CAD build for the part. Positions are in the model's coordinates, mm. A direction names the side the tool comes from. Round coordinates to 2 decimals unless told otherwise and drop trailing zeros. Order: outer loops, then holes, each group sorted by start corner. A loop starts at its lowest first (then second) coordinate and runs counter-clockwise, first axis right, second up. Notation, with made-up numbers: (81.5, -32) -> (93.5, -32) arc R31 ccw to (93.5, -1) -> close; hole circle Ø4 at (68.5, 47). An arc over 180 degrees is marked (long way). Return JSON: item names as keys, results as strings. Group by question number.
Q1. Which spindle directions (+Z, -Z, +X, -X, +Y, -Y) get a long thin tool onto all of the face, cutting with end or side? Do faces 4 (the flat face through (-31.18, -9, 2)), 5 (the flat face through (-31.18, 3, 5)), 6 (the flat face through (-37, 7.69, 5)). Say none if no direction does.
Q2. Cut at C-C (x = -12.5). Write the cut outline in (y, z), then the cut area to 3 significant figures.
Q3. Cut at D-D (y = -19). Write the cut outline in (x, z), then the cut area to 3 significant figures.
Q4. Cut at A-A (y = -3.5). Write the cut outline in (x, z).
Q5. Mould opens along X. For faces 1 (the flat face through (49.58, 22, 5)), 2 (the flat face through (24, 23, 9.35)), 3 (the flat face through (-2, 39.74, 3)) say: +X half, -X half, draft (parallel to the pull), parting line (faces both ways), or undercut.
Q6. Probe line 1 along X through (y, z) = (3, 4.75); line 2 along X through (y, z) = (6, 7); line 3 along X through (y, z) = (-5.5, 0.75). List the from-to ranges inside material, lowest first.
Q7. Flat gauge pins, fed straight in: pin 1 (5 mm diameter, centred on x = -64.5, z = 4, fed in from +Y); pin 2 (19 mm diameter, centred on x = -20.5, y = -2, fed in from +Z); pin 3 (1.6 mm diameter, centred on x = -10.5, z = 1, fed in from -Y). Where does each tip first touch, or does it go through?
Autodesk Inventor part; units mm, degrees
ref_plane "YZ Plane" through (0, 0, 0) normal (1, 0, 0) x (0, 1, 0)
ref_plane "XZ Plane" through (0, 0, 0) normal (0, 1, 0) x (-1, 0, 0)
ref_plane "XY Plane" through (0, 0, 0) normal (0, 0, 1) x (1, 0, 0)
sketch "Sketch1" plane through (0, 0, 0) normal (0, 0, 1) x (1, 0, 0)
  line L0 (0, 0) -> (49.58, 0)
  line L1 (49.58, 0) -> (49.58, 44.9)
  line L2 (49.58, 44.9) -> (0, 44.9)
  line L3 (0, 44.9) -> (0, 0)
  line L4 (49.58, 2.33) -> (27.13, 2.33)
  line L5 (27.13, 2.33) -> (27.13, 0)
  line L6 (27.13, 44.9) -> (27.13, 42.57)
  line L7 (27.13, 42.57) -> (49.58, 42.57)
  dimension "d0" = 49.58
  dimension "d1" = 44.9
  dimension "d2" = 22.45
  dimension "d3" = 2.33
extrude "Extrusion1" add sketch "Sketch1" along normal blind 9.35 contours L3 L2 L6 L7 L1 L4 L5 L0
sketch "Sketch2" plane through (0, 0, 0) normal (-1, 0, 0) x (0, 0, 1)
  line L0 (0, 44.9) -> (0, 0)
  line L1 (9.35, 44.9) -> (9.35, 0)
  line L2 (0, 44.9) -> (9.35, 44.9)
  line L3 (0, 39.74) -> (9.35, 39.74)
  line L4 (9.35, 39.74) -> (9.35, 7.69)
  line L5 (9.35, 7.69) -> (0, 7.69)
  line L6 (0, 7.69) -> (0, 39.74)
  dimension "d6" = 32.05
  dimension "d7" = 5.16
extrude "Extrusion2" add sketch "Sketch2" along normal blind 31.18 contours L3 L1 L5 L0
sketch "Sketch3" plane through (0, 0, 9.35) normal (0, 0, 1) x (1, 0, 0)
  line L0 (0, 39.74) -> (-31.18, 39.74)
  line L1 (-3.12, 39.74) -> (0, 39.74)
  line L2 (0, 39.74) -> (0, 7.69)
  line L3 (0, 7.69) -> (-3.12, 7.69)
  line L4 (-3.12, 7.69) -> (-3.12, 39.74)
extrude "Extrusion3" cut sketch "Sketch3" against normal blind 3.12
sketch "Sketch4" plane through (-31.18, 39.74, 0) normal (0, 1, 0) x (1, 0, 0)
  line L0 (0, -9.35) -> (0, 0)
  line L1 (28.06, -9.35) -> (0, -9.35)
  line L2 (31.18, 0) -> (0, 0)
  line L3 (28.06, -9.35) -> (0, -9.35)
  line L4 (0, -9.35) -> (0, 0)
  line L5 (0, 0) -> (28.06, 0)
  line L6 (28.06, 0) -> (28.06, -9.35)
extrude "Extrusion4" add sketch "Sketch4" along normal blind 6.86
sketch "Sketch5" plane through (-31.18, 7.69, 0) normal (0, -1, 0) x (1, 0, 0)
  line L0 (28.06, 0) -> (0, 0)
  line L1 (28.06, 9.35) -> (28.06, 0)
  line L2 (0, 0) -> (28.06, 0)
  line L3 (28.06, 0) -> (28.06, 3.12)
  line L4 (28.06, 3.12) -> (0, 3.12)
  line L5 (0, 3.12) -> (0, 0)
  dimension "d14" = 3.12
extrude "Extrusion5" add sketch "Sketch5" along normal blind 24.01
sketch "Sketch6" plane through (-31.18, 7.69, 3.12) normal (0, 0, 1) x (1, 0, 0)
  line L0 (0, 0) -> (9.35, 0)
  line L1 (9.35, 0) -> (9.35, -9.35)
  line L2 (9.35, -9.35) -> (0, -9.35)
  line L3 (0, -9.35) -> (0, 0)
  point P0 (31.18, -7.69)
  dimension "d17" = 9.35
  dimension "d18" = 9.35
extrude "Extrusion6" add sketch "Sketch6" along normal blind 3.12
sketch "Sketch7" plane through (-31.18, 0, 0) normal (-1, 0, 0) x (0, 0, 1)
  line L0 (3.12, 7.69) -> (0, 7.69)
  line L1 (3.12, -1.66) -> (0, -1.66)
  line L2 (0, -1.66) -> (0, 7.69)
  line L3 (0, 7.69) -> (3.12, 7.69)
  line L4 (3.12, 7.69) -> (3.12, -1.66)
  line L5 (0, 7.69) -> (6.24, 7.69)
  line L6 (6.24, 7.69) -> (6.24, 35.13)
  line L7 (6.24, 35.13) -> (0, 35.13)
  line L8 (0, 35.13) -> (0, 7.69)
  line L9 (0, -16.32) -> (0, 46.6)
  point P0 (0, 0)
  dimension "d21" = 27.44
  dimension "d24" = 6.24
extrude "Extrusion7" add sketch "Sketch7" along normal blind 12.47
sketch "Sketch8" plane through (-31.18, 35.13, 6.24) normal (0, 1, 0) x (1, 0, 0)
  line L0 (-12.47, 0) -> (-12.47, 6.24)
  line L1 (0, 6.24) -> (-12.47, 6.24)
  line L2 (0, 0) -> (-12.47, 0)
  line L3 (0, 6.24) -> (-3.12, 6.24)
  line L4 (-3.12, 6.24) -> (-3.12, 0)
  line L5 (-3.12, 0) -> (0, 0)
  line L6 (0, 0) -> (0, 6.24)
  point P0 (31.18, 6.24)
  dimension "d25" = 3.12
extrude "Extrusion8" cut sketch "Sketch8" against normal blind 6.24 contours L0 L1 L4 L2
sketch "Sketch9" plane through (-43.65, 0, 0) normal (-1, 0, 0) x (0, 0, 1)
  line L0 (0, 28.89) -> (0, -1.66)
  line L1 (0, 28.58) -> (9.35, 28.58)
  line L2 (9.35, 28.58) -> (9.35, -1.66)
  line L3 (9.35, -1.66) -> (0, -1.66)
  line L4 (0, -1.66) -> (0, 28.58)
  point P0 (0, 0)
extrude "Extrusion9" add sketch "Sketch9" along normal blind 28.06
sketch "Sketch10" plane through (-71.71, 0, 0) normal (-1, 0, 0) x (0, 0, 1)
  line L0 (0, 28.58) -> (0, -1.66)
  line L1 (0, 7.69) -> (6.24, 7.69)
  line L2 (6.24, 7.69) -> (6.24, -31.6)
  line L3 (6.24, -31.6) -> (0, -31.6)
  line L4 (0, -31.6) -> (0, 7.69)
  point P0 (0, 0)
  dimension "d30" = 39.29
extrude "Extrusion10" add sketch "Sketch10" along normal blind 23.7
sketch "Sketch11" plane through (-71.71, 0, 0) normal (1, 0, 0) x (0, 0, -1)
  line L0 (0, -1.66) -> (-6.24, -1.66)
  line L1 (-6.24, -1.66) -> (-6.24, -31.6)
  line L2 (-6.24, -31.6) -> (0, -31.6)
  line L3 (0, -31.6) -> (0, -1.66)
  point P0 (0, 0)
extrude "Extrusion11" add sketch "Sketch11" along normal blind 8.73
sketch "Sketch12" plane through (-62.98, 0, 0) normal (1, 0, 0) x (0, 0, -1)
  line L0 (0, -1.66) -> (-3.12, -1.66)
  line L1 (-3.12, -1.66) -> (-3.12, -28.48)
  line L2 (-3.12, -28.48) -> (0, -28.48)
  line L3 (0, -28.48) -> (0, -1.66)
  point P0 (0, 0)
  dimension "d35" = 26.82
extrude "Extrusion12" add sketch "Sketch12" along normal blind 19.33
sketch "Sketch13" plane through (-43.65, 0, 0) normal (1, 0, 0) x (0, 0, -1)
  line L0 (0, -28.48) -> (-6.24, -28.48)
  line L1 (-6.24, -28.48) -> (-6.24, -24.11)
  line L2 (-6.24, -24.11) -> (0, -24.11)
  line L3 (0, -24.11) -> (0, -28.48)
  point P0 (0, 0)
  dimension "d38" = 6.24
  dimension "d39" = 4.37
extrude "Extrusion13" add sketch "Sketch13" along normal blind 4.37
properties part number "Sportcenter" material "UHMW, White"
Solution:
{
 "1": {"face 4": "+Z, -Z, -Y", "face 5": "+Z, -Y", "face 6": "+Z"},
 "2": {"outline": "(-16.32, 0) -> (46.6, 0) -> (46.6, 9.35) -> (7.69, 9.35) -> (7.69, 3.12) -> (-16.32, 3.12) -> close", "area": "439 mm²"},
 "3": {"outline": "(-95.41, 0) -> (-43.65, 0) -> (-43.65, 3.12) -> (-62.98, 3.12) -> (-62.98, 6.24) -> (-95.41, 6.24) -> close", "area": "263 mm²"},
 "4": {"outline": "(-95.41, 0) -> (-43.65, 0) -> (-43.65, 3.12) -> (-62.98, 3.12) -> (-62.98, 6.24) -> (-95.41, 6.24) -> close; (-31.18, 0) -> (-3.12, 0) -> (-3.12, 3.12) -> (-31.18, 3.12) -> close"},
 "5": {"face 1": "+X half", "face 2": "draft", "face 3": "undercut"},
 "6": {"line 1": "x = -95.41 to -43.65, -31.18 to -21.83, 0 to 49.58", "line 2": "x = -71.71 to -43.65, 0 to 49.58", "line 3": "x = -95.41 to -43.65, -31.18 to -3.12"},
 "7": {"pin 1": "stops at y = 28.58", "pin 2": "stops at z = 6.24", "pin 3": "stops at y = -16.32"}
}
